Verification items for the finished model (mm, model axes). Round coordinates to 2 decimals unless told otherwise and drop trailing zeros. Write each loop counter-clockwise with the first axis right and the second up, starting at its lowest first coordinate (ties: lowest second). Pieces come first, ordered by that corner, then holes. Notation, with made-up numbers: (36.25, 87.5) - (85.25, 87.5) arc R20 cw to (85.25, 119.5) - close; hole circle Ø5 at (10.5, 85). An arc over 180 degrees is marked (long way). Answer as a JSON object with one key per item and string values. Group by question number.
1) Thickness scan on line 1 (Z direction, x = -0.8, y = -0.1); line 2 (Y direction, x = -1.25, z = 7.75); line 3 (Z direction, x = 1.7, y = 0.8). Record the ranges inside material, lowest first.
2) Section check A-A (x = 1.25). Enter the section's corners in (y, z).
3) Section check B-B (z = 1.75). Enter the section's corners in (x, y), then the cut area to 3 significant figures.
4) Mould release check, pull along X, two halves, no side actions. Record for faces 1 (the flat face through (0, 0, 5)), 2 (the flat face through (-2, 0, 2)), 3 (the flat face through (0, 1, 2)): +X half, -X half, draft (parallel to the pull), parting line (faces both ways), or undercut.
5) Go/stop test with flat-tipped pins: pin 1 Ø1 at (y, z) = (-1, 5.5) entering from -X; pin 2 Ø1 at (x, z) = (1.5, 9.5) entering from +Y. Record where each tip stops, or that it passes through.
6) Section check D-D (z = 13.5). Enter the section's corners in (x, y).
```python
from build123d import *

# Parameters (mm, degrees)
SKETCH1_W           = 4
SKETCH1_H           = 2
BOSS_EXTRUDE1_DEPTH = 5
SKETCH2_R           = 0.25
BOSS_EXTRUDE2_DEPTH = 10
FILLET1_R           = 0.5


with BuildPart() as part:
    # Sketch1 → Boss-Extrude1 (new body)
    with BuildSketch(Plane.XY):
        Rectangle(SKETCH1_W, SKETCH1_H)
    extrude(amount=BOSS_EXTRUDE1_DEPTH)

    # Sketch2 → Boss-Extrude2 (add)
    with BuildSketch(Plane.XY.offset(5)):
        with Locations(Location((-1.25, 0, 0), (0, 0, 180))):
            Circle(SKETCH2_R)
        with Locations(Location((1.25, 0, 0), (0, 0, 180))):
            Circle(SKETCH2_R)
    extrude(amount=BOSS_EXTRUDE2_DEPTH)

    # Fillet1
    fillet1_edges = [part.edges().sort_by_distance(p)[0] for p in [
        (-2, 0, 5),
        (0, -1, 5),
        (2, 0, 5),
        (0, -1, 0),
        (-2, 0, 0),
        (0, 1, 0),
        (2, 0, 0),
        (0, 1, 5),
        (2, -1, 2.5),
        (-2, -1, 2.5),
        (-2, 1, 2.5),
        (2, 1, 2.5),
    ]]
    fillet(fillet1_edges, radius=FILLET1_R - 0.0001)  # a hair under: the kernel refuses the full size


solid = part.part
```
Returned:
{
 "1": {"line 1": "0 to 5", "line 2": "-0.25 to 0.25", "line 3": "0.15 to 4.85"},
 "2": {"outline": "(-1, 0.5) arc R0.5 ccw to (-0.5, 0) - (0.5, 0) arc R0.5 ccw to (1, 0.5) - (1, 4.5) arc R0.5 ccw to (0.5, 5) - (0.25, 5) - (0.25, 15) - (-0.25, 15) - (-0.25, 5) - (-0.5, 5) arc R0.5 ccw to (-1, 4.5) - close"},
 "3": {"outline": "(-2, -0.5) arc R0.5 ccw to (-1.5, -1) - (1.5, -1) arc R0.5 ccw to (2, -0.5) - (2, 0.5) arc R0.5 ccw to (1.5, 1) - (-1.5, 1) arc R0.5 ccw to (-2, 0.5) - close", "area": "7.79 mm2"},
 "4": {"face 1": "undercut", "face 2": "-X half", "face 3": "draft"},
 "5": {"pin 1": "through", "pin 2": "y = 0.25"},
 "6": {"outline": "circle Ø0.5 at (-1.25, 0); circle Ø0.5 at (1.25, 0)"}
}
